Geometry: final body of the model. Coordinates: model frame, mm. A direction names the side the tool comes from. Give positions to 0.01 mm unless a question says otherwise; leave off trailing zeros. Write each loop counter-clockwise with the first axis right and the second up, starting at its lowest first coordinate (ties: lowest second). Pieces come first, ordered by that corner, then holes.
```python
from build123d import *

# Parameters (mm, degrees)
SKETCH_1_R          = 23.1
EXTRUDE_1_DEPTH     = 2
SKETCH_2_R          = 23.1
SKETCH_2_R_2        = 21.05
EXTRUDE_2_DEPTH     = 13
SKETCH_3_R          = 4
CUT_EXTRUDE_1_DEPTH = 36.159920364


with BuildPart() as part:
    # 草图1 → 凸台-拉伸1 (new body)
    with BuildSketch(Plane(origin=(0, 0, 0), x_dir=(1, 0, 0), z_dir=(0, 1, 0))):
        with Locations(Location((0, 0, 0), (0, 0, 270))):
            Circle(SKETCH_1_R)
    extrude(amount=EXTRUDE_1_DEPTH)

    # 草图2 → 凸台-拉伸2 (add)
    with BuildSketch(Plane(origin=(0, 2, 0), x_dir=(1, 0, 0), z_dir=(0, 1, 0))):
        with Locations(Location((0, 0, 0), (0, 0, 270))):
            Circle(SKETCH_2_R)
        with Locations(Location((0, 0, 0), (0, 0, 90))):
            Circle(SKETCH_2_R_2, mode=Mode.SUBTRACT)
    extrude(amount=EXTRUDE_2_DEPTH)

    # 草图3 → 切除-拉伸1 (cut, through all)
    with BuildSketch(Plane(origin=(0, 2, 0), x_dir=(1, 0, 0), z_dir=(0, 1, 0))):
        with Locations(Location((0, 0, 0), (0, 0, 270))):
            Circle(SKETCH_3_R)
    extrude(amount=-CUT_EXTRUDE_1_DEPTH, mode=Mode.SUBTRACT)


solid = part.part
```
Item 1: Section C-C, the plane y = 11.5. Return the cut outline in (x, z), plus the area to 3 significant figures.
Found:
outline: circle Ø46.2 at (0, 0); hole circle Ø42.1 at (0, 0)
area: 284 mm2
Item 2: Section A-A, the plane z = 0. Return the cut outline in (x, y).
Found:
outline: (-23.1, 0) - (-4, 0) - (-4, 2) - (-21.05, 2) - (-21.05, 15) - (-23.1, 15) - close; (4, 0) - (23.1, 0) - (23.1, 15) - (21.05, 15) - (21.05, 2) - (4, 2) - close
Item 3: Section B-B, the plane x = 0. Return the cut outline in (y, z).
Found:
outline: (0, -23.1) - (15, -23.1) - (15, -21.05) - (2, -21.05) - (2, -4) - (0, -4) - close; (0, 4) - (2, 4) - (2, 21.05) - (15, 21.05) - (15, 23.1) - (0, 23.1) - close
Item 4: Pin query (flat end, axial travel): pin 1 Ø1 at (x, y) = (-16, 2.5) entering from +Z; pin 2 Ø9 at (x, z) = (0, 0) entering from +Y; pin 3 Ø3 at (y, z) = (4.5, -18) entering from -X. Return the tip coordinate at first contact, or that it passes through.
Found:
pin 1: stops at z = 17.13
pin 2: stops at y = 2
pin 3: stops at x = -16.17
Item 5: Section D-D, the plane z = 10. Return the cut outline in (x, y), plus the area to 3 significant figures.
Found:
outline: (-20.82, 0) - (20.82, 0) - (20.82, 15) - (18.52, 15) - (18.52, 2) - (-18.52, 2) - (-18.52, 15) - (-20.82, 15) - close
area: 143 mm2
Item 6: Line query: L1, parallel to X at y = 12, z = 0; L2, parallel to X at y = 1.1, z = 0; L3, parallel to Y at x = -12.5, z = -15. Output: solid intervals per line, ascending.
Found:
L1: x = -23.1 to -21.05, 21.05 to 23.1
L2: x = -23.1 to -4, 4 to 23.1
L3: y = 0 to 2
Item 7: Pull-direction query (X, two-part tool) for faces 3 (the face through (-19, 15, 10)), 4 (the face through (-22.55, 7.4, -5.01)), 5 (the face through (-4.4, 2, -0.3)); classes: +X half, -X half, draft (parallel to the pull), parting line (faces both ways), or undercut.
Found:
face 3: draft
face 4: parting line
face 5: undercut
Item 8: Reachability of faces 1 (the face through (0, 0, 5)), 2 (the face through (8.062, 8.409, -19.445)) from +Z, -Z, +X, -X, +Y, -Y: full face, straight path, thin tool, end or side. Return the list, or none.
Found:
face 1: +Z, -Z, +X, -X, -Y
face 2: +Y
